```python
from build123d import *

# Parameters (mm, degrees)
F0_W     = 63.5
F0_H     = 38.1
F1_DEPTH = 25.4
F2_R     = 12.7
F3_DEPTH = 25.4


with BuildPart() as f1:
    # F0 (on Front) → F1 (new body)
    with BuildSketch(Plane.XZ):
        Polygon((40.64, 68.58), (0, 38.1), (63.5, 38.1), align=None)
        with Locations((31.75, 19.05)):
            Rectangle(F0_W, F0_H)
    extrude(amount=F1_DEPTH)

    # F2 (on face) → F3 (join)
    with BuildSketch(Plane.XZ.offset(25.4)):
        Polygon((63.5, 38.1), (40.64, 68.58), (0, 38.1), (0, 0), (63.5, 0), align=None)
        with Locations((38.1, 25.4)):
            Circle(F2_R, mode=Mode.SUBTRACT)
    extrude(amount=F3_DEPTH)


solid = f1.part
```
The model under review builds one solid part; all positions refer to its coordinate system, in mm. A direction names the side the tool comes from. Round coordinates to 2 decimals unless told otherwise and drop trailing zeros. Loops run counter-clockwise (first coordinate to the right, second up) from the corner with the lowest first, then second, coordinate; pieces in that order, holes last. Notation, with made-up numbers: M -6.75,-32.5 L 47.25,-32.5 A34 ccw 47.25,-0.5 Z; hole C 87,14 d1. An arc over 180 degrees is marked long. Put each result on its own line as item: value.
Q1. Consider section A-A, the plane z = 25.4. Give the boundary of the cut face in (x, y).
Result set:
outline: M 0,-50.8 L 25.4,-50.8 L 25.4,-25.4 L 50.8,-25.4 L 50.8,-50.8 L 63.5,-50.8 L 63.5,0 L 0,0 Z
Q2. For pin 1 (1 mm diameter, centred on y = -30, z = 54, fed in from +X); pin 2 (12 mm diameter, centred on x = 46.5, y = -22, fed in from +Z); pin 3 (2 mm diameter, centred on y = -20, z = 45, fed in from +X) (3 decimals), all flat-tipped, find the tip position at first contact; note any pin that passes through.
Result set:
pin 1: stops at x = 51.95
pin 2: stops at z = 68.58
pin 3: stops at x = 59.075
Q3. Consider section C-C, the plane x = 38.1. Give the boundary of the cut face in (y, z) (3 decimals).
Result set:
outline: M -50.8,0 L 0,0 L 0,66.675 L -50.8,66.675 L -50.8,38.1 L -25.4,38.1 L -25.4,12.7 L -50.8,12.7 Z
Q4. Mouldability with a two-part tool opening along Z and no side actions: class faces 1 (the cylindrical face through (44.927, -37.922, 36.109)), 2 (the flat face through (63.5, -25, 19)), 3 (the flat face through (52.23, -25.04, 53.13)) as released by +Z, released by -Z, zero draft, split by the parting line, or undercut.
Result set:
face 1: undercut
face 2: zero draft
face 3: released by +Z
Q5. Consider section B-B, the plane y = -46.5. Give the boundary of the cut face in (x, z).
Result set:
outline: M 0,0 L 63.5,0 L 63.5,38.1 L 40.64,68.58 L 0,38.1 Z; hole C 38.1,25.4 d25.4
Q6. Machinability: for faces 4 (the flat face through (31, 0, 27)), 5 (the flat face through (38, -25.4, 26)), which of the approach directions +Z, -Z, +X, -X, +Y, -Y give a long, thin tool a straight path to every point of the face, cutting with its end or side? Answer none if there is none.
Result set:
face 4: +Z, -Z, +X, -X, +Y
face 5: -Y
Q7. To check wall thickness, follow L1, parallel to X at y = -34, z = 25; L2, parallel to Z at x = 28, y = -36.5; L3, parallel to Z at x = 38.5, y = -39.5 (3 decimals). State the ranges of each line that lie inside material, in increasing order.
Result set:
L1: x = 0 to 25.41, 50.79 to 63.5
L2: z = 0 to 17.7, 33.1 to 59.1
L3: z = 0 to 12.706, 38.094 to 66.975
Q8. Consider section D-D, the plane y = -24. Give the boundary of the cut face in (x, z), then the cut area to 3 significant figures.
Result set:
outline: M 0,0 L 63.5,0 L 63.5,38.1 L 40.64,68.58 L 0,38.1 Z
area: 3,390 mm²
